Part model, mm, in its own coordinate system. Give positions to 0.01 mm unless a question says otherwise; leave off trailing zeros. Write each loop counter-clockwise with the first axis right and the second up, starting at its lowest first coordinate (ties: lowest second). Pieces come first, ordered by that corner, then holes. Notation, with made-up numbers: (-21, -39.75) - (-12, -39.75) arc R21 cw to (-12, -0.75) - close; hole circle Ø1 at (15, 70). An arc over 180 degrees is marked (long way). Answer as a JSON object with one key per item and string values. Group by question number.
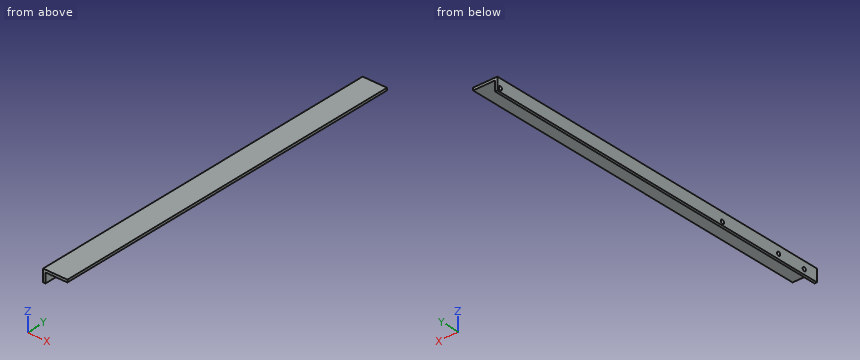
```python
from build123d import *

# Parameters (mm, degrees)
BOSS_EXTRUDE1_DEPTH      = 300
SKETCH2_R                = 1.5
CUT_EXTRUDE1_DEPTH       = 301.83217913
F_3_0_3_DIAMETER_HOLE1_D = 3


with BuildPart() as part:
    # Sketch1 → Boss-Extrude1 (new body)
    with BuildSketch(Plane(origin=(0, 0, 0), x_dir=(1, 0, 0), z_dir=(0, 1, 0))):
        Polygon((0, 0), (0, 10), (2, 10), (2, 2), (20, 2), (20, 0), align=None)
    extrude(amount=BOSS_EXTRUDE1_DEPTH)

    # Sketch2 → Cut-Extrude1 (cut, through all)
    with BuildSketch(Plane.ZY):
        with Locations((-7.262612197, 297.245406858)):
            Circle(SKETCH2_R)
        with Locations((-7.258467028, 88.743438507)):
            Circle(SKETCH2_R)
    extrude(amount=-CUT_EXTRUDE1_DEPTH, mode=Mode.SUBTRACT)

    # Ø3.0 (3) Diameter Hole1 (through all)
    with Locations(Plane(origin=(2, -25.407632793, 52.861996081), x_dir=(0, 0, -1), z_dir=(1, 0, 0))):
        with Locations((58.861996081, 61.407632793), (58.861996081, 37.407632793)):
            Hole(F_3_0_3_DIAMETER_HOLE1_D / 2)


solid = part.part
```
1) Drill centre lines: line 1 along Y through (x, z) = (1, -6); line 2 along Y through (x, z) = (1.25, -8.25); line 3 along X through (y, z) = (117, -8.5). Where is each one in solid material? Low to high. Write a range as from..to.
2) Drop flat-ended pins along their axis: P1, Ø2.5, axis at y = 88.74, z = -7.26, coming from the -X side; P2, Ø2.5, axis at y = 76.5, z = -7.5, coming from the +X side. Give the stop position or say it passes through.
3) Saw through at A-A (x = 12.5). List the corners of the cut face in (y, z), and give its area (3 significant figures).
4) Saw through at B-B (y = 152.5). List the corners of the cut face in (x, z).
Checks:
{
 "1": {"line 1": "0..10.5, 13.5..34.5, 37.5..87.93, 89.56..296.44, 298.06..300", "line 2": "0..87.62, 89.87..296.12, 298.37..300", "line 3": "0..2"},
 "2": {"P1": "through", "P2": "x = 2"},
 "3": {"outline": "(0, -2) - (300, -2) - (300, 0) - (0, 0) - close", "area": "600 mm2"},
 "4": {"outline": "(0, -10) - (2, -10) - (2, -2) - (20, -2) - (20, 0) - (0, 0) - close"}
}
